Autodesk Inventor part; units mm, degrees
ref_plane "YZ Plane" through (0, 0, 0) normal (1, 0, 0) x (0, 1, 0)
ref_plane "XZ Plane" through (0, 0, 0) normal (0, 1, 0) x (-1, 0, 0)
ref_plane "XY Plane" through (0, 0, 0) normal (0, 0, 1) x (1, 0, 0)
sketch "スケッチ1" plane through (0, 0, 0) normal (0, 0, 1) x (1, 0, 0)
  circle A0 centre (0, 0) radius 65 construction
  line L0 (-42.5, 65) -> (42.5, 65) construction
  line L1 (42.5, 65) -> (42.5, -65) construction
  line L2 (42.5, -65) -> (-42.5, -65) construction
  line L3 (-42.5, -65) -> (-42.5, 65) construction
  arc A1 (42.5, 49.1808) -> (-42.5, 49.1808) centre (0, 0) ccw
  line L4 (-42.5, 49.1808) -> (-42.5, -49.1808)
  line L5 (42.5, 49.1808) -> (42.5, -49.1808)
  arc A2 (-42.5, -49.1808) -> (42.5, -49.1808) centre (0, 0) ccw
  point P0 (0, 65)
  dimension "d0" = 130
  dimension "d1" = 85
extrude "基板" add sketch "スケッチ1" along normal blind 1.6
sketch "スケッチ2" plane through (0, 0, 1.6) normal (0, 0, 1) x (1, 0, 0)
  line L0 (-100.8621, 0) -> (100.8621, 0) construction
  line L1 (0, 110.7931) -> (0, -110.7931) construction
  line L2 (-42.5, 49.1808) -> (-42.5, -49.1808) construction
  circle A0 centre (0, 0) radius 60 construction
  point P0 (-36.5, 9)
  point P1 (-30.5, 9)
  point P2 (30.5, 9)
  point P3 (36.5, 9)
  point P4 (-36.5, -9)
  point P5 (-30.5, -9)
  point P6 (30.5, -9)
  point P7 (36.5, -9)
  point P8 (-40, -30)
  point P9 (-40, -45)
  point P10 (-42.5, -49.1808)
  point P11 (-27.5, -17.5)
  point P12 (-27.5, 17.5)
  point P13 (27.5, -17.5)
  point P14 (27.5, 17.5)
  dimension "d4" = 18
  dimension "d5" = 6
  dimension "d6" = 6
  dimension "d26" = 120
  dimension "d38" = 35
  dimension "d39" = 15
hole "モータ取付穴" at (-36.5, 9, 1.6) at (-30.5, 9, 1.6) at (30.5, 9, 1.6) at (36.5, 9, 1.6) at (-36.5, -9, 1.6) at (-30.5, -9, 1.6) at (30.5, -9, 1.6) at (36.5, -9, 1.6) at (-27.5, -17.5, 1.6) at (-27.5, 17.5, 1.6) at (27.5, -17.5, 1.6) at (27.5, 17.5, 1.6) direction (0, 0, -1) diameter 2.1 end through all
sketch "スケッチ3" plane through (0, 0, 1.6) normal (0, 0, 1) x (1, 0, 0)
  line L0 (0, 0) -> (0, 55.332) construction
  line L1 (-15.38, 55) -> (15.38, 55) construction
  line L2 (0, 46.85) -> (-7.0581, 50.925) construction
  line L3 (-7.0581, 50.925) -> (-7.0581, 59.075) construction
  line L4 (-7.0581, 59.075) -> (0, 63.15) construction
  line L5 (0, 63.15) -> (7.0581, 59.075) construction
  line L6 (7.0581, 59.075) -> (7.0581, 50.925) construction
  line L7 (7.0581, 50.925) -> (0, 46.85) construction
  arc A0 (42.5, 49.1808) -> (-42.5, 49.1808) centre (0, 0) ccw construction
  point P0 (0, 55)
  point P1 (0, 55)
  point P2 (0, 65)
  dimension "d17" = 16.3
  dimension "d18" = 10
hole "ボールキャスター取付穴" at (-7.0581, 59.075, 1.6) at (7.0581, 59.075, 1.6) at (0, 46.85, 1.6) direction (0, 0, -1) diameter 3.2 end through all
sketch "スケッチ4" plane through (0, 0, 1.6) normal (0, 0, 1) x (1, 0, 0)
  line L0 (0, -55.1622) -> (0, 55.1622) construction
  line L1 (42.5, -49.1808) -> (42.5, 49.1808) construction
  circle A0 centre (0, 0) radius 60 construction
  line L2 (0, 0) -> (36.3616, 43.334) construction
  line L3 (0, 0) -> (56.5685, 0) construction
  point P0 (38.5, -46.019)
  point P1 (-38.5, -46.019)
  point P2 (38.5673, 45.9627)
  point P3 (-38.5673, 45.9627)
  dimension "d27" = 4
  dimension "d29" = 120
  dimension "d30" = 50
hole "スペーサ取付穴" at (38.5, -46.019, 1.6) at (-38.5, -46.019, 1.6) at (38.5673, 45.9627, 1.6) at (-38.5673, 45.9627, 1.6) direction (0, 0, -1) diameter 3.2 end through all
mirror "ミラー1" about plane through (0, 0, 0) normal (0, 1, 0) of "ボールキャスター取付穴"
properties part number "BaseBoard2"
Build history of the part. All positions in model axes, mm. Round coordinates to 2 decimals unless told otherwise and drop trailing zeros. Write each loop counter-clockwise with the first axis right and the second up, starting at its lowest first coordinate (ties: lowest second). Pieces come first, ordered by that corner, then holes.
1) Pin check, flat tip, straight feed: pin 1 (1.3 mm diameter, centred on x = -30.5, y = 9, fed in from +Z). Stop position of the tip, or through.
2) Band-saw the part on B-B, the plane z = 1. Give the number of separate pieces and of enclosed holes in the cut face, and give its area (3 significant figures).
3) Band-saw the part on C-C, the plane x = -33. List the corners of the cut face in (y, z), and give its area (3 significant figures).
4) Band-saw the part on A-A, the plane x = 0. List the corners of the cut face in (y, z).
5) Mould opens along X. For faces 1 (the cylindrical face through (-0.649, 64.997, 0.789)), 2 (the flat face through (-1, 1, 0)), 3 (the cylindrical face through (-0.481, 45.324, 0.789)) say: +X half, -X half, draft (parallel to the pull), parting line (faces both ways), or undercut.
6) Drill centre lines: probe 1 along X at (y, z) = (9, 1.3); probe 2 along Y at (x, z) = (38, 0.45); probe 3 along Y at (x, z) = (31, 0.8). Where is each one in solid material? Low to high.
Ans:
1. pin 1: passes through
2. separate pieces: 1
2. enclosed holes: 22
2. area: 10,100 mm2
3. outline: (-56, 0) - (56, 0) - (56, 1.6) - (-56, 1.6) - close
3. area: 179 mm2
4. outline: (-65, 0) - (-48.45, 0) - (-48.45, 1.6) - (-65, 1.6) - close; (-45.25, 0) - (45.25, 0) - (45.25, 1.6) - (-45.25, 1.6) - close; (48.45, 0) - (65, 0) - (65, 1.6) - (48.45, 1.6) - close
5. face 1: parting line
5. face 2: draft
5. face 3: undercut
6. probe 1: x = -42.5 to -37.55, -35.45 to -31.55, -29.45 to 29.45, 31.55 to 35.45, 37.55 to 42.5
6. probe 2: y = -52.74 to -47.54, -44.5 to 44.47, 47.46 to 52.74
6. probe 3: y = -57.13 to -9.92, -8.08 to 8.08, 9.92 to 57.13
